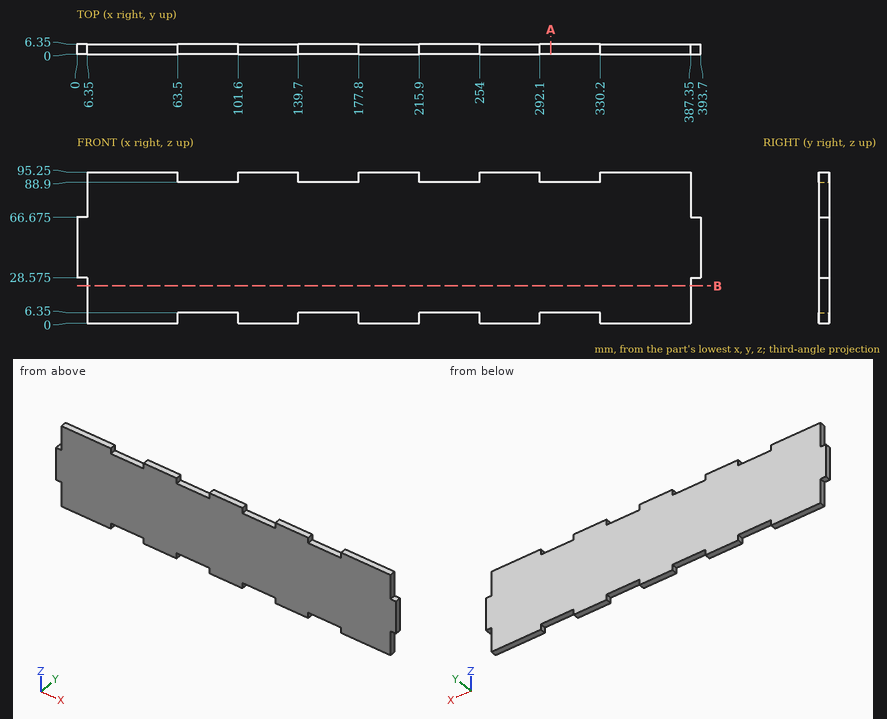
Verification items for this drawing (mm, ordinates from the low corner). Round coordinates to 2 decimals unless told otherwise and drop trailing zeros. Write each loop counter-clockwise with the first axis right and the second up, starting at its lowest first coordinate (ties: lowest second). Pieces come first, ordered by that corner, then holes. Notation, with made-up numbers: (14, 40.5) - (19, 40.5) arc R31 cw to (19, 76.5) - close; hole circle Ø3 at (86.5, 16.25). An arc over 180 degrees is marked (long way). Answer as a JSON object with one key per item and string values. Group by question number.
Q1. Go/stop test with flat-tipped pins: pin 1 Ø3 at (x, y) = (310, 3) entering from +Z; pin 2 Ø8 at (x, z) = (148.5, 25.5) entering from -Y; pin 3 Ø3 at (y, z) = (2, 4.5) entering from -X; pin 4 Ø3 at (y, z) = (3, 93.5) entering from +X. Record where each tip stops, or that it passes through.
Q2. Section check A-A, the plane x = 299. Enter the section's corners in (y, z).
Q3. Section check B-B, the plane z = 23.5. Enter the section's corners in (x, y).
Q4. Thickness scan on line 1 (X direction, y = 5.5, z = 90.5); line 2 (Z direction, x = 317.5, y = 1.5); line 3 (X direction, y = 2, z = 86). Record the ranges inside material, lowest first.
Found:
{
 "1": {"pin 1": "stops at z = 88.9", "pin 2": "stops at y = 0", "pin 3": "stops at x = 6.35", "pin 4": "stops at x = 387.35"},
 "2": {"outline": "(0, 6.35) - (6.35, 6.35) - (6.35, 88.9) - (0, 88.9) - close"},
 "3": {"outline": "(6.35, 0) - (387.35, 0) - (387.35, 6.35) - (6.35, 6.35) - close"},
 "4": {"line 1": "x = 6.35 to 63.5, 101.6 to 139.7, 177.8 to 215.9, 254 to 292.1, 330.2 to 387.35", "line 2": "z = 6.35 to 88.9", "line 3": "x = 6.35 to 387.35"}
}
